CAD build for the part. Positions are in the model's coordinates, mm. A direction names the side the tool comes from. Round coordinates to 2 decimals unless told otherwise and drop trailing zeros. Loops run counter-clockwise (first coordinate to the right, second up) from the corner with the lowest first, then second, coordinate; pieces in that order, holes last. Notation, with made-up numbers: (-10, 77.25) -> (42, 77.25) arc R20 ccw to (42, 97.25) -> close; hole circle Ø7 at (-31, 72). An arc over 180 degrees is marked (long way). Answer as CSV lines item,"result".
```python
from build123d import *

# Parameters (mm, degrees)
F0_W     = 1000
F0_H     = 500
F1_DEPTH = 25.4
F2_W     = 25
F2_H     = 25
F3_DEPTH = 530
F5_DEPTH = 3


with BuildPart() as f1:
    # F0 (on Top) → F1 (new body)
    with BuildSketch(Plane.XY):
        Rectangle(F0_W, F0_H)
    extrude(amount=F1_DEPTH)

    # F2 (on face) → F3 (join)
    with BuildSketch(Plane(origin=(0, 0, 0), x_dir=(1, 0, 0), z_dir=(0, 0, -1))):
        with Locations((-487.5, 237.5)):
            Rectangle(F2_W, F2_H)
        with Locations((-487.5, -237.5)):
            Rectangle(F2_W, F2_H)
        with Locations((487.5, 237.5)):
            Rectangle(F2_W, F2_H)
        with Locations((487.5, -237.5)):
            Rectangle(F2_W, F2_H)
    extrude(amount=F3_DEPTH)

    # F4 (on face) → F5 (join)
    with BuildSketch(Plane(origin=(0, 250, 0), x_dir=(-1, 0, 0), z_dir=(0, 1, 0))):
        with BuildLine():
            Line((-500, 119.05), (-500, 25.4))
            Line((-500, 25.4), (500, 25.4))
            Line((500, 25.4), (500, 119.05))
            ThreePointArc((500, 119.05), (498.140128, 123.540128), (493.65, 125.4))
            Line((493.65, 125.4), (-493.65, 125.4))
            ThreePointArc((-493.65, 125.4), (-498.140128, 123.540128), (-500, 119.05))
        make_face()
    extrude(amount=-F5_DEPTH)


solid = f1.part
```
Q1. Tool access for faces 4 (the flat face through (-7, 2, 25.4)), 5 (the flat face through (-475, -237, -261)), 6 (the flat face through (487, 225, -261)): list every direction of +Z, -Z, +X, -X, +Y, -Y with a clear straight run to the whole face (end or side of a thin tool).
Results:
face 4,"+Z, +X, -X, -Y"
face 5,"-Z, +Y, -Y"
face 6,"-Z, +X, -X"
Q2. Probe L1, parallel to X at y = -225.5, z = -383; L2, parallel to Z at x = -29.5, y = -127.5; L3, parallel to Y at x = -182, z = 66. List the from-to ranges inside material, lowest first. Write a range as [from, to].
Results:
L1,"[-500, -475], [475, 500]"
L2,"[0, 25.4]"
L3,"[247, 250]"
Q3. Slice it at C-C, the plane x = -301.5. Give the cut face in (y, z), and give its area (3 significant figures).
Results:
outline,"(-250, 0) -> (250, 0) -> (250, 125.4) -> (247, 125.4) -> (247, 25.4) -> (-250, 25.4) -> close"
area,"13,000 mm2"
Q4. Drop flat-ended pins along their axis: pin 1 Ø10 at (x, y) = (364, -150.5) entering from +Z; pin 2 Ø3 at (x, y) = (-113, -154) entering from -Z. Give the stop position or say it passes through.
Results:
pin 1,"z = 25.4"
pin 2,"z = 0"
Q5. Two-plate mould, pull along Y, no slides. Class faces 1 (the flat face through (-488, -225, -261)), 2 (the flat face through (475, -237, -261)), 3 (the flat face through (7, 247, 76)): pulls with the +Y half, pulls with the -Y half, needs draft (parallel to the pull), parting line crosses it, or undercut.
Results:
face 1,"undercut"
face 2,"needs draft"
face 3,"pulls with the -Y half"
Q6. Slice it at A-A, the plane z = -23. Give the cut face in (x, y).
Results:
outline,"(-500, -250) -> (-475, -250) -> (-475, -225) -> (-500, -225) -> close; (-500, 225) -> (-475, 225) -> (-475, 250) -> (-500, 250) -> close; (475, -250) -> (500, -250) -> (500, -225) -> (475, -225) -> close; (475, 225) -> (500, 225) -> (500, 250) -> (475, 250) -> close"
Q7. Slice it at B-B, the plane y = -86. Give the cut face in (x, z).
Results:
outline,"(-500, 0) -> (500, 0) -> (500, 25.4) -> (-500, 25.4) -> close"
Q8. Slice it at D-D, the plane z = 84.5. Give the cut face in (x, y).
Results:
outline,"(-500, 247) -> (500, 247) -> (500, 250) -> (-500, 250) -> close"
